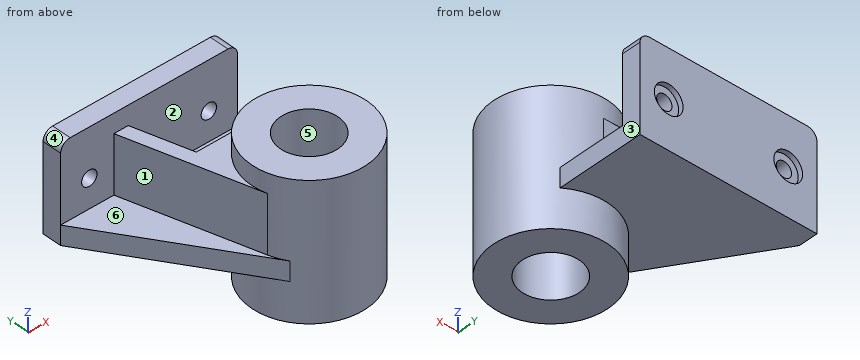
from build123d import *

# Parameters (mm, degrees)
SKETCH1_R                                 = 60
SKETCH1_R_2                               = 30
BOSS_EXTRUDE1_DEPTH                       = 70
BOSS_EXTRUDE4_DEPTH                       = 60
BOSS_EXTRUDE5_DEPTH                       = 20
BOSS_EXTRUDE6_DEPTH                       = 20
CBORE_FOR_M12_HEX_HEAD_SCREW1_D           = 16
CBORE_FOR_M12_HEX_HEAD_SCREW1_DEPTH       = 20
CBORE_FOR_M12_HEX_HEAD_SCREW1_CBORE_D     = 30
CBORE_FOR_M12_HEX_HEAD_SCREW1_CBORE_DEPTH = 5
CBORE_FOR_M12_HEX_HEAD_SCREW1_TIP         = 4.806884952


with BuildPart() as part:
    # Sketch1 → Boss-Extrude1 (new body, symmetric)
    with BuildSketch(Plane.XY):
        Circle(SKETCH1_R)
        Circle(SKETCH1_R_2, mode=Mode.SUBTRACT)
    extrude(amount=BOSS_EXTRUDE1_DEPTH, both=True)

    # Sketch4 → Boss-Extrude4 (add)
    with BuildSketch(Plane.XY.offset(50)):
        with BuildLine():
            Line((-94.270473916, 120), (-79.270473916, 120))
            Line((-79.270473916, 120), (-63.19352237, 60))
            Line((-63.19352237, 60), (0, 60))
            ThreePointArc((0, 60), (-47.601200417, 36.525685741), (-57.955549577, -15.529142706))
            Line((-57.955549577, -15.529142706), (-94.270473916, 120))
        make_face()
    extrude(amount=-BOSS_EXTRUDE4_DEPTH)

    # Sketch7 → Boss-Extrude5 (add)
    with BuildSketch(Plane(origin=(0, 0, -10), x_dir=(-1, 0, 0), z_dir=(0, 0, -1))):
        with BuildLine():
            Line((150, 120), (-35, 120))
            Line((-35, 120), (-35, 48.733971724))
            ThreePointArc((-35, 48.733971724), (41.47341809, 43.358454676), (50.240561153, -32.800701441))
            Line((50.240561153, -32.800701441), (150, 120))
        make_face()
    extrude(amount=BOSS_EXTRUDE5_DEPTH)

    # Sketch8 → Boss-Extrude6 (add)
    with BuildSketch(Plane(origin=(0, 120, 0), x_dir=(1, 0, 0), z_dir=(0, 1, 0))):
        with BuildLine():
            Line((-150, 30), (-150, -60))
            ThreePointArc((-150, -60), (-147.071067812, -67.071067812), (-140, -70))
            Line((-140, -70), (25, -70))
            ThreePointArc((25, -70), (32.071067812, -67.071067812), (35, -60))
            Line((35, -60), (35, 30))
            Line((35, 30), (-150, 30))
        make_face()
    extrude(amount=BOSS_EXTRUDE6_DEPTH)

    # CBORE for M12 Hex Head Screw1
    with Locations(Plane(origin=(0, 140, 0), x_dir=(1, 0, 0), z_dir=(0, 1, 0))):
        with Locations((-120, -20), (5, -20)):
            CounterBoreHole(CBORE_FOR_M12_HEX_HEAD_SCREW1_D / 2, CBORE_FOR_M12_HEX_HEAD_SCREW1_CBORE_D / 2, CBORE_FOR_M12_HEX_HEAD_SCREW1_CBORE_DEPTH, depth=CBORE_FOR_M12_HEX_HEAD_SCREW1_DEPTH)
            with Locations((0, 0, -(CBORE_FOR_M12_HEX_HEAD_SCREW1_DEPTH + CBORE_FOR_M12_HEX_HEAD_SCREW1_TIP / 2))):  # 118° drill point
                Cone(0, CBORE_FOR_M12_HEX_HEAD_SCREW1_D / 2, CBORE_FOR_M12_HEX_HEAD_SCREW1_TIP, mode=Mode.SUBTRACT)


solid = part.part
Could you check a few things on this model? Use its own coordinates, in mm. Face numbers are marked on the shaded views. A direction names the side the tool comes from. Coordinates: 2 decimals unless noted, no trailing zeros. Order: outer loops, then holes, each group sorted by start corner. A loop starts at its lowest first (then second) coordinate and runs counter-clockwise, first axis right, second up.
Q1. Please list where these lines run through material, in increasing order: L1, parallel to Y at x = 0, z = 26.5; L2, parallel to Z at x = -120, y = 124.25; L3, parallel to Z at x = -120, y = 138.55.
Q2. Suppose I cut it at D-D on z = -20. Please give me the cut outline in (x, y), and give its area (3 significant figures).
Q3. Suppose I cut it at A-A on z = 20. Please give me the cut outline in (x, y).
Q4. Which directions (+Z, -Z, +X, -X, +Y, -Y) give clear straight access to the entire face, cutting with the end or side of a thin tool? Please do the marked faces 1, 2 and 3.
Q5. Thinking about a two-plate mould opening in X: for the marked faces 4, 5 and 6, which applies, released by +X, released by -X, zero draft, split by the parting line, or undercut?
Q6. Suppose I cut it at C-C on x = -120. Please give me the cut outline in (y, z), and give its area (3 significant figures).
Q7. Suppose I cut it at B-B on y = 0. Please give me the cut outline in (x, z).
Q8. Will these pins go through, and if not, where does the flat tip stop? pin 1 (3 mm diameter, centred on y = 52.5, z = 52, fed in from +X); pin 2 (15 mm diameter, centred on x = 5, z = 15.5, fed in from +Y); pin 3 (1.5 mm diameter, centred on x = -105, y = 79.5, fed in from -Z).
Answer:
1. L1: y = -60 to -30, 30 to 60, 120 to 135
1. L2: z = -30 to 12, 28 to 70
1. L3: z = -30 to 5, 35 to 70
2. outline: (-150, 120) - (-50.24, -32.8) arc R60 ccw (long way) to (35, 48.73) - (35, 140) - (-150, 140) - close; hole circle Ø60 at (0, 0)
2. area: 25,000 mm2
3. outline: (-150, 120) - (-128, 120) - (-128, 135) - (-135, 135) - (-135, 140) - (-150, 140) - close; (-112, 120) - (-94.27, 120) - (-57.96, -15.53) arc R60 ccw (long way) to (0, 60) - (-63.19, 60) - (-79.27, 120) - (-3, 120) - (-3, 135) - (-10, 135) - (-10, 140) - (-105, 140) - (-105, 135) - (-112, 135) - close; (13, 120) - (35, 120) - (35, 140) - (20, 140) - (20, 135) - (13, 135) - close; hole circle Ø60 at (0, 0)
4. face 1: +Z, -X, -Y
4. face 2: +Z
4. face 3: +Z, -Z, +X, +Y
5. face 4: released by -X
5. face 5: undercut
5. face 6: zero draft
6. outline: (74.05, -30) - (140, -30) - (140, 5) - (135, 5) - (135, 12) - (120, 12) - (120, -10) - (74.05, -10) - close; (120, 28) - (135, 28) - (135, 35) - (140, 35) - (140, 70) - (120, 70) - close
6. area: 2,530 mm2
7. outline: (-71.66, -30) - (-60, -30) - (-60, -70) - (-30, -70) - (-30, 70) - (-60, 70) - (-60, 50) - (-62.12, 50) - (-62.12, -10) - (-71.66, -10) - close; (30, -70) - (60, -70) - (60, 70) - (30, 70) - close
8. pin 1: stops at x = 31.61
8. pin 2: stops at y = 135
8. pin 3: stops at z = -30
